from build123d import *

# Parameters (mm, degrees)
SKETCH_1_R          = 17.6
SKETCH_1_R_2        = 2.5
EXTRUDE_1_DEPTH     = 36
EXTRUDE_START       = -2
SKETCH_1_4_R        = 2.5
EXTRUDE_2_DEPTH     = 2
EXTRUDE_START_2     = 36
SKETCH_1_5_R        = 2.5
EXTRUDE_3_DEPTH     = 18.5
SKETCH_2_R          = 1.5
CUT_EXTRUDE_1_DEPTH = 3


with BuildPart() as part:
    # Эскиз1 → Бобышка-Вытянуть1 (new body)
    # profile 1 of 2: a face of its own
    with BuildSketch(Plane.XY):
        Circle(SKETCH_1_R)
        Circle(SKETCH_1_R_2, mode=Mode.SUBTRACT)
    # profile 2 of 2: a face of its own
    with BuildSketch(Plane.XY):
        Circle(SKETCH_1_R_2)
    extrude(amount=EXTRUDE_1_DEPTH)

    # Эскиз1<4> → Бобышка-Вытянуть2 (add)
    with BuildSketch(Plane.XY.offset(EXTRUDE_START)):
        Circle(SKETCH_1_4_R)
    extrude(amount=EXTRUDE_2_DEPTH)

    # Эскиз1<5> → Бобышка-Вытянуть3 (add)
    with BuildSketch(Plane.XY.offset(EXTRUDE_START_2)):
        Circle(SKETCH_1_5_R)
    extrude(amount=EXTRUDE_3_DEPTH)

    # Эскиз2 → Вырез-Вытянуть1 (cut)
    with BuildSketch(Plane(origin=(0, 0, 0), x_dir=(-1, 0, 0), z_dir=(0, 0, -1))):
        with Locations((0, 12.5)):
            Circle(SKETCH_2_R)
        with Locations((-9.5, 0)):
            Circle(SKETCH_2_R)
        with Locations(Location((0, -12.5, 0), (0, 0, 180))):
            Circle(SKETCH_2_R)
        with Locations(Location((9.5, 0, 0), (0, 0, 180))):
            Circle(SKETCH_2_R)
    extrude(amount=-CUT_EXTRUDE_1_DEPTH, mode=Mode.SUBTRACT)


solid = part.part
The model under review builds one solid part; all positions refer to its coordinate system, in mm. A direction names the side the tool comes from. Give positions to 0.01 mm unless a question says otherwise; leave off trailing zeros. Loops run counter-clockwise (first coordinate to the right, second up) from the corner with the lowest first, then second, coordinate; pieces in that order, holes last. Notation, with made-up numbers: (-1.5, -17.5) -> (47.5, -17.5) arc R20 cw to (47.5, -2.5) -> close; hole circle Ø5 at (75, 77.25). An arc over 180 degrees is marked (long way). Answer as a JSON object with one key per item and string values. Group by question number.
Q1. Insertion check: pin 1 (5 mm diameter, centred on x = -2, y = -8, fed in from +Z); pin 2 (1.5 mm diameter, centred on x = -0.5, y = -13, fed in from -Z); pin 3 (5 mm diameter, centred on y = 11.5, z = 25.5, fed in from -X). Each pin has a flat end and moves straight along its axis. Give the tip position at first contact, or say it passes through.
Q2. Take a section at C-C (z = 26). Write out the cut boundary in (x, y), plus the area to 3 significant figures.
Q3. Take a section at B-B (x = 0). Write out the cut boundary in (y, z).
Q4. Take a section at D-D (y = -12.5). Write out the cut boundary in (x, z), plus the area to 3 significant figures.
Q5. Take a section at A-A (y = 0). Write out the cut boundary in (x, z).
Q6. Draft analysis for pull direction Y (two halves, no side actions). For faces 4 (the cylindrical face through (-11, 0, 1)), 5 (the flat face through (0, 13, 3)), 6 (the flat face through (4, 0, 0)), 7 (the cylindrical face through (16.787, 5.287, 17.748)), state which applies: pulls with the +Y half, pulls with the -Y half, needs draft (parallel to the pull), parting line crosses it, or undercut.
Q7. Tool access review of faces 1 (the cylindrical face through (0, 11, 1)), 2 (the cylindrical face through (-0.54, -2.44, 45.12)), 3 (the flat face through (0, 0, -2)): name each direction out of +Z, -Z, +X, -X, +Y, -Y from which nothing blocks a thin tool from reaching the whole face with its end or side.
Q8. Wall thickness on line 1 along Y through (x, z) = (0, 1); line 2 along Z through (x, y) = (-7, 6); line 3 along Y through (x, z) = (0, 42.5): over which ranges is each line inside the solid? List them lowest first.
Answer below:
{
 "1": {"pin 1": "stops at z = 36", "pin 2": "stops at z = 3", "pin 3": "stops at x = -15.12"},
 "2": {"outline": "circle Ø35.2 at (0, 0)", "area": "973 mm2"},
 "3": {"outline": "(-17.6, 0) -> (-14, 0) -> (-14, 3) -> (-11, 3) -> (-11, 0) -> (-2.5, 0) -> (-2.5, -2) -> (2.5, -2) -> (2.5, 0) -> (11, 0) -> (11, 3) -> (14, 3) -> (14, 0) -> (17.6, 0) -> (17.6, 36) -> (2.5, 36) -> (2.5, 54.5) -> (-2.5, 54.5) -> (-2.5, 36) -> (-17.6, 36) -> close"},
 "4": {"outline": "(-12.39, 0) -> (-1.5, 0) -> (-1.5, 3) -> (1.5, 3) -> (1.5, 0) -> (12.39, 0) -> (12.39, 36) -> (-12.39, 36) -> close", "area": "883 mm2"},
 "5": {"outline": "(-17.6, 0) -> (-11, 0) -> (-11, 3) -> (-8, 3) -> (-8, 0) -> (-2.5, 0) -> (-2.5, -2) -> (2.5, -2) -> (2.5, 0) -> (8, 0) -> (8, 3) -> (11, 3) -> (11, 0) -> (17.6, 0) -> (17.6, 36) -> (2.5, 36) -> (2.5, 54.5) -> (-2.5, 54.5) -> (-2.5, 36) -> (-17.6, 36) -> close"},
 "6": {"face 4": "undercut", "face 5": "undercut", "face 6": "needs draft", "face 7": "parting line crosses it"},
 "7": {"face 1": "-Z", "face 2": "+Z", "face 3": "-Z, +X, -X, +Y, -Y"},
 "8": {"line 1": "y = -17.6 to -14, -11 to 11, 14 to 17.6", "line 2": "z = 0 to 36", "line 3": "y = -2.5 to 2.5"}
}
